Autodesk Inventor part; units mm, degrees
ref_plane "作業平面3" through (135, 0, 0) normal (1, 0, 0) x (0, 1, 0)
ref_plane "XZ Plane" through (0, 0, 0) normal (0, 1, 0) x (-1, 0, 0)
ref_plane "XY Plane" through (0, 0, 0) normal (0, 0, 1) x (1, 0, 0)
sketch "Sketch_2" plane through (0, 0, 0) normal (0, 0, 1) x (1, 0, 0)
  arc A0 (-20, 13.3) -> (-20, -13.3) centre (-20, 0) ccw
  line L0 (-20, -13.3) -> (290, -13.3)
  arc A1 (290, -13.3) -> (290, 13.3) centre (290, 0) ccw
  line L1 (290, 13.3) -> (-20, 13.3)
extrude "Extrusion1" add sketch "Sketch_2" along normal mid plane 20
sketch "Sketch_8" plane through (0, 0, 0) normal (0, 0, 1) x (1, 0, 0)
  line L0 (-1.5, 28.3) -> (-1.5, 13.3)
  line L1 (-1.5, 13.3) -> (1.5, 13.3)
  line L2 (1.5, 13.3) -> (1.5, 28.3)
  line L3 (1.5, 28.3) -> (-1.5, 28.3)
extrude "Extrusion2" add sketch "Sketch_8" along normal mid plane 19
sketch "_____4" plane through (0, 0, 0) normal (1, 0, 0) x (0, 0, -1)
  circle A0 centre (-4.5, 22.3) radius 2.25
extrude "Extrusion3" cut sketch "_____4" along normal mid plane 6
sketch "_____5" plane through (0, 0, 0) normal (1, 0, 0) x (0, 0, -1)
  circle A0 centre (4.5, 22.3) radius 2.25
extrude "Extrusion4" cut sketch "_____5" along normal mid plane 6
sketch "_____2" plane through (0, 0, 0) normal (0, 0, 1) x (1, 0, 0)
  line L0 (33.5, 8.3) -> (36.5, 8.3)
  line L1 (36.5, 8.3) -> (36.5, 28.3)
  line L2 (36.5, 28.3) -> (33.5, 28.3)
  line L3 (33.5, 28.3) -> (33.5, 8.3)
extrude "Extrusion5" add sketch "_____2" along normal mid plane 19
sketch "Sketch6" plane through (33.5, 13.3, 9.5) normal (-1, 0, 0) x (0, 0, 1)
  point P0 (-14, 9)
hole "Hole1" at (33.5, 22.3, -4.5) direction (1, 0, 0) diameter 4.5 depth 3
sketch "Sketch7" plane through (33.5, 13.3, 9.5) normal (-1, 0, 0) x (0, 0, 1)
  point P0 (-5, 9)
hole "Hole2" at (33.5, 22.3, 4.5) direction (1, 0, 0) diameter 4.5 depth 3
sketch "Sketch_4" plane through (0, 0, 0) normal (0, 0, 1) x (1, 0, 0)
  arc A0 (-20, 12.3) -> (-20, -12.3) centre (-20, 0) ccw
  line L0 (-20, -12.3) -> (290, -12.3)
  arc A1 (290, -12.3) -> (290, 12.3) centre (290, 0) ccw
  line L1 (290, 12.3) -> (17.5, 12.3)
  line L2 (17.5, 12.3) -> (17.5, 11.1)
  line L3 (17.5, 11.1) -> (-7.5, 11.1)
  line L4 (-7.5, 11.1) -> (-7.5, 12.3)
  line L5 (-7.5, 12.3) -> (-20, 12.3)
extrude "Extrusion6" cut sketch "Sketch_4" along normal mid plane 20
sketch "Sketch_64" plane through (0, 0, 0) normal (0, 0, 1) x (1, 0, 0)
  line L0 (-9.3801, 11.1) -> (-9.3801, 10.1)
  line L1 (-9.3801, 10.1) -> (-5.6199, 10.1)
  line L2 (-5.6199, 10.1) -> (-5.6199, 11.1)
  arc A0 (-5.9958, 11.3632) -> (-5.6199, 11.1) centre (-5.6199, 11.5) ccw
  line L3 (-5.9958, 11.3632) -> (-6.241, 12.0368)
  arc A1 (-6.241, 12.0368) -> (-6.6168, 12.3) centre (-6.6168, 11.9) ccw
  line L4 (-6.6168, 12.3) -> (-7.125, 12.3)
  line L5 (-7.125, 12.3) -> (-7.125, 12.66)
  line L6 (-7.125, 12.66) -> (-7.875, 12.66)
  line L7 (-7.875, 12.66) -> (-7.875, 12.3)
  line L8 (-7.875, 12.3) -> (-8.3832, 12.3)
  arc A2 (-8.3832, 12.3) -> (-8.759, 12.0368) centre (-8.3832, 11.9) ccw
  line L9 (-8.759, 12.0368) -> (-9.0042, 11.3632)
  arc A3 (-9.3801, 11.1) -> (-9.0042, 11.3632) centre (-9.3801, 11.5) ccw
extrude "Extrusion7" cut sketch "Sketch_64" along normal mid plane 20
pattern_linear "Rectangular Pattern1" count 6 spacing 5 along (1, 0, 0) of "Extrusion7"
ref_plane "作業平面3" through (135, 0, 0) normal (1, 0, 0) x (0, 1, 0)
ref_plane "作業平面1" through (303.3, 0, 0) normal (1, 0, 0) x (0, 1, 0)
ref_plane "作業平面2" through (-33.3, 0, 0) normal (1, 0, 0) x (0, 1, 0)
properties part number "ATBT-700T5200-B-P35_info-1-16-16"
Geometry: final body of the model. Coordinates: model frame, mm. A direction names the side the tool comes from. Round coordinates to 2 decimals unless told otherwise and drop trailing zeros. Write each loop counter-clockwise with the first axis right and the second up, starting at its lowest first coordinate (ties: lowest second). Pieces come first, ordered by that corner, then holes. Notation, with made-up numbers: (31.5, 29.25) -> (35.5, 29.25) arc R18 ccw to (35.5, 47.25) -> close; hole circle Ø8 at (16.25, -21.75). An arc over 180 degrees is marked (long way). Use CSV: the item, a comma, the result in double quotes. Start each with the question number.
Q1. Reachability of faces 5 (the face through (33.5, 21, 0)), 6 (the face through (-1.5, 21, 0)), 7 (the face through (-32.297, -0.27, -0.14)) from +Z, -Z, +X, -X, +Y, -Y: full face, straight path, thin tool, end or side. Return the list, or none.
Q2. Section B-B (x = 169). Return loops of the section in (y, z).
Q3. Line query: L1, parallel to Z at x = -0.55, y = 22.3; L2, parallel to Y at x = -0.25, z = 4.5; L3, parallel to Y at x = 35.3, z = -4.5. Output: solid intervals per line, ascending.
Q4. Section A-A (y = 17). Return loops of the section in (x, z).
Q5. Pull-direction query (X, two-part tool) for faces 1 (the face through (36.5, 21, 0)), 2 (the face through (1.5, 21, 0)), 3 (the face through (134, 13, 10)), 4 (the face through (302.297, 0.27, -0.14)); classes: pulls with the +X half, pulls with the -X half, needs draft (parallel to the pull), parting line crosses it, or undercut.
Q6. First-contact query: pin 1 Ø7.5 at (y, z) = (23, 1) entering from +X; pin 2 Ø1 at (y, z) = (2.5, -7.5) entering from -X; pin 3 Ø5 at (y, z) = (22.3, 4.5) entering from -X. Flat tips, straight axial feed; report the tip coordinate or a pass-through.
Result sheet:
1,face 5,"+Z, -Z, +Y"
1,face 6,"+Z, -Z, -X, +Y"
1,face 7,"+Z, -Z"
2,outline,"(-13.3, -10) -> (-12.3, -10) -> (-12.3, 10) -> (-13.3, 10) -> close; (12.3, -10) -> (13.3, -10) -> (13.3, 10) -> (12.3, 10) -> close"
3,L1,"-9.5 to -6.75, -2.25 to 2.25, 6.75 to 9.5"
3,L2,"-13.3 to -12.3, 11.1 to 20.05, 24.55 to 28.3"
3,L3,"-13.3 to -12.3, 12.3 to 20.05, 24.55 to 28.3"
4,outline,"(-1.5, -9.5) -> (1.5, -9.5) -> (1.5, 9.5) -> (-1.5, 9.5) -> close; (33.5, -9.5) -> (36.5, -9.5) -> (36.5, 9.5) -> (33.5, 9.5) -> close"
5,face 1,"pulls with the +X half"
5,face 2,"undercut"
5,face 3,"needs draft"
5,face 4,"undercut"
6,pin 1,"x = 36.5"
6,pin 2,"x = -33.15"
6,pin 3,"x = -1.5"
